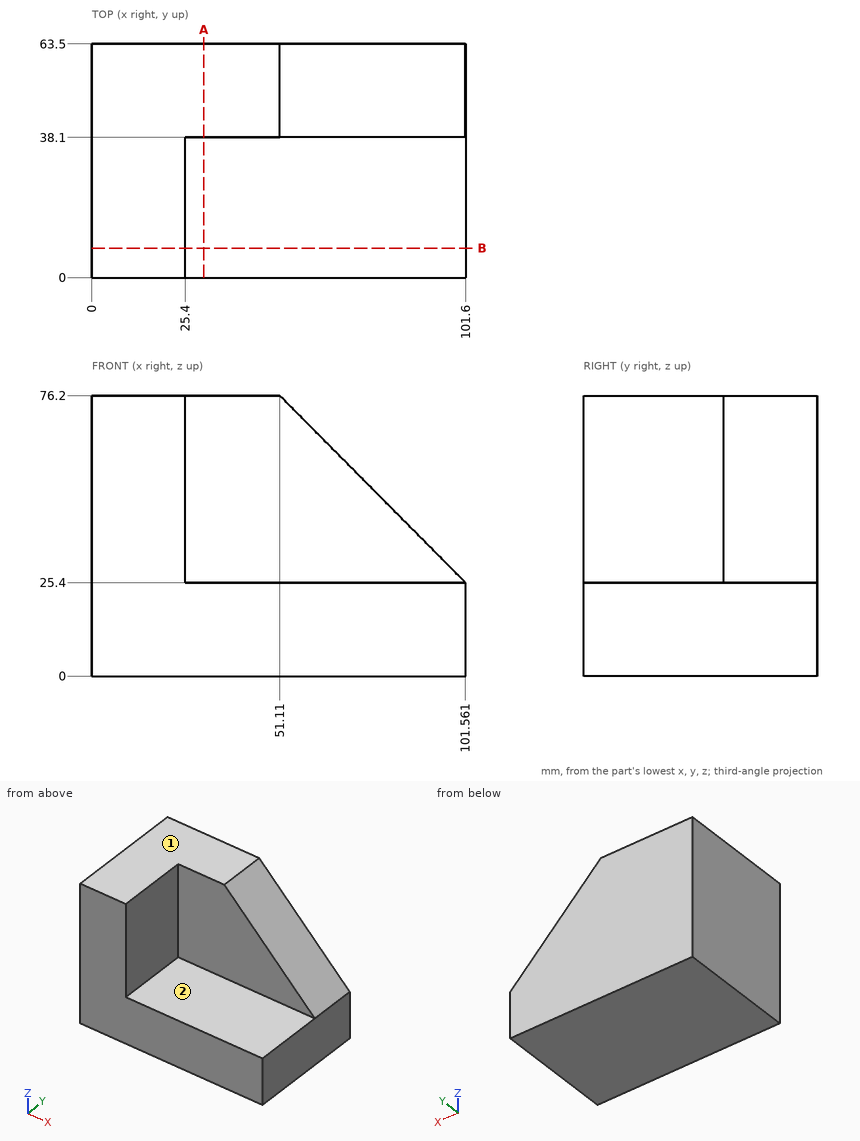
The drawing under review shows one solid part. Ordinate dimensions are in mm from its lowest x, y, z. A direction names the side the tool comes from. Round coordinates to 2 decimals unless told otherwise and drop trailing zeros. Loops run counter-clockwise (first coordinate to the right, second up) from the corner with the lowest first, then second, coordinate; pieces in that order, holes last. Notation, with made-up numbers: (17, 48.5) - (76, 48.5) arc R10 cw to (76, 67.5) - close; hole circle Ø8 at (-21.75, -32.5). An arc over 180 degrees is marked (long way). Put each result on its own line as item: value. Start each with the question number.
1. Consider section A-A on x = 30.5. State the section outline as (y, z) points, plus the area to 3 significant figures.
2. For probe 1 along X at (y, z) = (30.5, 56.5); probe 2 along Y at (x, z) = (53, 59.5), list the stretches that pass through material, from the lowest coordinate up. Write a range as [from, to].
3. Insertion check: P1, Ø6, axis at x = 40.5, z = 23.5, coming from the -Y side; P2, Ø1, axis at x = 29, y = 30.5, coming from the +Z side; P3, Ø8, axis at y = 40.5, z = 58.5, coming from the +X side. Each pin has a flat end and moves straight along its axis. Give the tip position at first contact, or say it passes through.
4. For the marked faces 1 and 2, list the 3-axis set-ups (+Z, -Z, +X, -X, +Y, -Y) from which the entire face can be reached by the end or side of a thin tool; tool diameter is ignored.
5. Consider section B-B on y = 8. State the section outline as (x, z) points.
Result sheet:
1. outline: (0, 0) - (63.5, 0) - (63.5, 76.2) - (38.1, 76.2) - (38.1, 25.4) - (0, 25.4) - close
1. area: 2,900 mm^2
2. probe 1: [0, 25.4]
2. probe 2: [38.1, 63.5]
3. P1: y = 0
3. P2: z = 25.4
3. P3: x = 72.66
4. face 1: +Z, +X, -X, +Y, -Y
4. face 2: +Z, +X, -Y
5. outline: (0, 0) - (101.6, 0) - (101.6, 25.4) - (25.4, 25.4) - (25.4, 76.2) - (0, 76.2) - close
